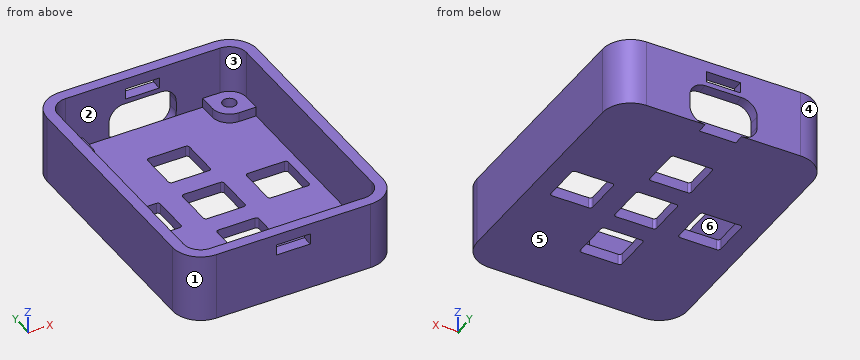
from build123d import *

# Parameters (mm, degrees)
BOX011_W          = 10
BOX011_H          = 3.2
BOX011_DEPTH      = 6.2
FILLET008_R       = 2.29
BOX013_W          = 5
BOX013_H          = 1.6
BOX013_DEPTH      = 1.6
BOX012_W          = 5
BOX012_H          = 1.6
BOX012_DEPTH      = 1.6
BOX009_W          = 6.2
BOX009_H          = 6.2
BOX009_DEPTH      = 2
FILLET004_R       = 0.4
BOX007_W          = 6.2
BOX007_H          = 6.2
BOX007_DEPTH      = 2
FILLET005_R       = 0.4
BOX010_W          = 6.2
BOX010_H          = 6.2
BOX010_DEPTH      = 2
FILLET006_R       = 0.4
BOX006_W          = 6.2
BOX006_H          = 6.2
BOX006_DEPTH      = 2
FILLET007_R       = 0.4
BOX008_W          = 6.2
BOX008_H          = 6.2
BOX008_DEPTH      = 2
FILLET003_R       = 0.4
CYLINDER003_R     = 1
CYLINDER003_DEPTH = 10
CYLINDER002_R     = 1
CYLINDER002_DEPTH = 10
CYLINDER001_R     = 1
CYLINDER001_DEPTH = 10
CYLINDER_R        = 1
CYLINDER_DEPTH    = 10
BOX002_W          = 5.08
BOX002_H          = 5.08
BOX002_DEPTH      = 3
BOX003_W          = 5.08
BOX003_H          = 5.08
BOX003_DEPTH      = 3
BOX004_W          = 5.08
BOX004_H          = 5.08
BOX004_DEPTH      = 3
BOX005_W          = 5.08
BOX005_H          = 5.08
BOX005_DEPTH      = 3
BOX001_W          = 28
BOX001_H          = 38.2
BOX001_DEPTH      = 10
BOX_W             = 31.2
BOX_H             = 41.4
BOX_DEPTH         = 10.1
FILLET_R          = 2.54
FILLET001_R       = 2.54
FILLET002_R       = 4.14


with BuildPart() as led:
    # Box011 → Box011 (new body)
    with BuildSketch(Plane(origin=(9, 38.2, 0), x_dir=(1, 0, 0), z_dir=(0, 0, 1))):
        with Locations((5, 1.6)):
            Rectangle(BOX011_W, BOX011_H)
    extrude(amount=BOX011_DEPTH)

    # Fillet008
    fillet008_edges = [led.edges().sort_by_distance(p)[0] for p in [
        (9, 39.8, 6.2),
        (9, 39.8, 0),
        (19, 39.8, 6.2),
        (19, 39.8, 0),
    ]]
    fillet(fillet008_edges, radius=FILLET008_R)


with BuildPart() as obj1:
    # Box013 → Box013 (new body)
    with BuildSketch(Plane(origin=(11.5, 38.2, 6.9), x_dir=(1, 0, 0), z_dir=(0, 0, 1))):
        with Locations((2.5, 0.8)):
            Rectangle(BOX013_W, BOX013_H)
    extrude(amount=BOX013_DEPTH)


with BuildPart() as nut:
    # Box012 → Box012 (new body)
    with BuildSketch(Plane(origin=(11.5, -1.6, 6.9), x_dir=(1, 0, 0), z_dir=(0, 0, 1))):
        with Locations((2.5, 0.8)):
            Rectangle(BOX012_W, BOX012_H)
    extrude(amount=BOX012_DEPTH)

    # Fusion003: union obj1
    add(obj1.part)


with BuildPart() as fillet004:
    # Box009 → Box009 (new body)
    with BuildSketch(Plane(origin=(1.4, 16.3, 0), x_dir=(1, 0, 0), z_dir=(0, 0, 1))):
        with Locations((3.1, 3.1)):
            Rectangle(BOX009_W, BOX009_H)
    extrude(amount=BOX009_DEPTH)

    # Fillet004
    fillet004_edges = [fillet004.edges().sort_by_distance(p)[0] for p in [
        (1.4, 16.3, 1),
        (1.4, 22.5, 1),
        (7.6, 16.3, 1),
        (7.6, 22.5, 1),
    ]]
    fillet(fillet004_edges, radius=FILLET004_R)


with BuildPart() as fillet005:
    # Box007 → Box007 (new body)
    with BuildSketch(Plane(origin=(10.9, 16.3, 0), x_dir=(1, 0, 0), z_dir=(0, 0, 1))):
        with Locations((3.1, 3.1)):
            Rectangle(BOX007_W, BOX007_H)
    extrude(amount=BOX007_DEPTH)

    # Fillet005
    fillet005_edges = [fillet005.edges().sort_by_distance(p)[0] for p in [
        (10.9, 16.3, 1),
        (10.9, 22.5, 1),
        (17.1, 16.3, 1),
        (17.1, 22.5, 1),
    ]]
    fillet(fillet005_edges, radius=FILLET005_R)


with BuildPart() as fillet006:
    # Box010 → Box010 (new body)
    with BuildSketch(Plane(origin=(20.4, 16.3, 0), x_dir=(1, 0, 0), z_dir=(0, 0, 1))):
        with Locations((3.1, 3.1)):
            Rectangle(BOX010_W, BOX010_H)
    extrude(amount=BOX010_DEPTH)

    # Fillet006
    fillet006_edges = [fillet006.edges().sort_by_distance(p)[0] for p in [
        (20.4, 16.3, 1),
        (20.4, 22.5, 1),
        (26.6, 16.3, 1),
        (26.6, 22.5, 1),
    ]]
    fillet(fillet006_edges, radius=FILLET006_R)


with BuildPart() as fillet007:
    # Box006 → Box006 (new body)
    with BuildSketch(Plane(origin=(10.9, 7.2, 0), x_dir=(1, 0, 0), z_dir=(0, 0, 1))):
        with Locations((3.1, 3.1)):
            Rectangle(BOX006_W, BOX006_H)
    extrude(amount=BOX006_DEPTH)

    # Fillet007
    fillet007_edges = [fillet007.edges().sort_by_distance(p)[0] for p in [
        (10.9, 7.2, 1),
        (10.9, 13.4, 1),
        (17.1, 7.2, 1),
        (17.1, 13.4, 1),
    ]]
    fillet(fillet007_edges, radius=FILLET007_R)


with BuildPart() as buttons:
    # Box008 → Box008 (new body)
    with BuildSketch(Plane(origin=(10.9, 25.5, 0), x_dir=(1, 0, 0), z_dir=(0, 0, 1))):
        with Locations((3.1, 3.1)):
            Rectangle(BOX008_W, BOX008_H)
    extrude(amount=BOX008_DEPTH)

    # Fillet003
    fillet003_edges = [buttons.edges().sort_by_distance(p)[0] for p in [
        (10.9, 25.5, 1),
        (10.9, 31.7, 1),
        (17.1, 25.5, 1),
        (17.1, 31.7, 1),
    ]]
    fillet(fillet003_edges, radius=FILLET003_R)

    # Fusion002: union Fillet004, Fillet005, Fillet006, Fillet007
    add(fillet004.part)
    add(fillet005.part)
    add(fillet006.part)
    add(fillet007.part)


with BuildPart() as zylinder003:
    # Cylinder003 → Cylinder003 (new body)
    with BuildSketch(Plane(origin=(25.46, 35.66, 0.4), x_dir=(1, 0, 0), z_dir=(0, 0, 1))):
        Circle(CYLINDER003_R)
    extrude(amount=CYLINDER003_DEPTH)


with BuildPart() as zylinder002:
    # Cylinder002 → Cylinder002 (new body)
    with BuildSketch(Plane(origin=(2.54, 35.66, 0.4), x_dir=(1, 0, 0), z_dir=(0, 0, 1))):
        Circle(CYLINDER002_R)
    extrude(amount=CYLINDER002_DEPTH)


with BuildPart() as zylinder001:
    # Cylinder001 → Cylinder001 (new body)
    with BuildSketch(Plane(origin=(25.46, 2.54, 0.4), x_dir=(1, 0, 0), z_dir=(0, 0, 1))):
        Circle(CYLINDER001_R)
    extrude(amount=CYLINDER001_DEPTH)


with BuildPart() as fusion001:
    # Cylinder → Cylinder (new body)
    with BuildSketch(Plane(origin=(2.54, 2.54, 0.4), x_dir=(1, 0, 0), z_dir=(0, 0, 1))):
        Circle(CYLINDER_R)
    extrude(amount=CYLINDER_DEPTH)

    # Fusion001: union Zylinder003, Zylinder002, Zylinder001
    add(zylinder003.part)
    add(zylinder002.part)
    add(zylinder001.part)


with BuildPart() as obj2:
    # Box002 → Box002 (new body)
    with BuildSketch(Plane.XY):
        with Locations((2.54, 2.54)):
            Rectangle(BOX002_W, BOX002_H)
    extrude(amount=BOX002_DEPTH)


with BuildPart() as obj3:
    # Box003 → Box003 (new body)
    with BuildSketch(Plane(origin=(22.92, 0, 0), x_dir=(1, 0, 0), z_dir=(0, 0, 1))):
        with Locations((2.54, 2.54)):
            Rectangle(BOX003_W, BOX003_H)
    extrude(amount=BOX003_DEPTH)


with BuildPart() as obj4:
    # Box004 → Box004 (new body)
    with BuildSketch(Plane(origin=(0, 33.12, 0), x_dir=(1, 0, 0), z_dir=(0, 0, 1))):
        with Locations((2.54, 2.54)):
            Rectangle(BOX004_W, BOX004_H)
    extrude(amount=BOX004_DEPTH)


with BuildPart() as obj5:
    # Box005 → Box005 (new body)
    with BuildSketch(Plane(origin=(22.92, 33.12, 0), x_dir=(1, 0, 0), z_dir=(0, 0, 1))):
        with Locations((2.54, 2.54)):
            Rectangle(BOX005_W, BOX005_H)
    extrude(amount=BOX005_DEPTH)


with BuildPart() as obj6:
    # Box001 → Box001 (new body)
    with BuildSketch(Plane.XY.offset(1.6)):
        with Locations((14, 19.1)):
            Rectangle(BOX001_W, BOX001_H)
    extrude(amount=BOX001_DEPTH)


with BuildPart() as cut005:
    # Box → Box (new body)
    with BuildSketch(Plane(origin=(-1.6, -1.6, 0), x_dir=(1, 0, 0), z_dir=(0, 0, 1))):
        with Locations((15.6, 20.7)):
            Rectangle(BOX_W, BOX_H)
    extrude(amount=BOX_DEPTH)

    # Cut: cut obj6
    add(obj6.part, mode=Mode.SUBTRACT)

    # Fusion: union obj2, obj3, obj4, obj5
    add(obj2.part)
    add(obj3.part)
    add(obj4.part)
    add(obj5.part)

    # Fillet
    fillet_edges = [cut005.edges().sort_by_distance(p)[0] for p in [
        (22.92, 33.12, 2.3),
        (22.92, 5.08, 2.3),
        (5.08, 33.12, 2.3),
        (5.08, 5.08, 2.3),
    ]]
    fillet(fillet_edges, radius=FILLET_R)

    # Fillet001
    fillet001_edges = [cut005.edges().sort_by_distance(p)[0] for p in [
        (28, 38.2, 6.55),
        (0, 38.2, 6.55),
        (28, 0, 6.55),
        (0, 0, 6.55),
    ]]
    fillet(fillet001_edges, radius=FILLET001_R)

    # Fillet002
    fillet002_edges = [cut005.edges().sort_by_distance(p)[0] for p in [
        (-1.6, -1.6, 5.05),
        (-1.6, 39.8, 5.05),
        (29.6, 39.8, 5.05),
        (29.6, -1.6, 5.05),
    ]]
    fillet(fillet002_edges, radius=FILLET002_R)

    # Cut001: cut Fusion001
    add(fusion001.part, mode=Mode.SUBTRACT)

    # Cut003: cut Buttons
    add(buttons.part, mode=Mode.SUBTRACT)

    # Cut004: cut Nut
    add(nut.part, mode=Mode.SUBTRACT)

    # Cut005: cut LED
    add(led.part, mode=Mode.SUBTRACT)


solid = cut005.part
The model under review builds one solid part; all positions refer to its coordinate system, in mm. Face numbers are marked on the shaded views. A direction names the side the tool comes from. Coordinates: 2 decimals unless noted, no trailing zeros. Write each loop counter-clockwise with the first axis right and the second up, starting at its lowest first coordinate (ties: lowest second). Pieces come first, ordered by that corner, then holes. Notation, with made-up numbers: (-14.5, 53) - (0.5, 53) arc R8 ccw to (0.5, 60) - close; hole circle Ø9 at (58.25, 53). An arc over 180 degrees is marked (long way). Answer as a JSON object with one key per item and string values. Group by question number.
1. Add section A-A (x = 12.5). Give the number of separate pieces and of enclosed holes in the cut face, plus the area to 3 significant figures.
2. Add section B-B (y = 10.5). Give the boundary of the cut face in (x, z).
3. Add section C-C (x = 21.5). Give the boundary of the cut face in (y, z), plus the area to 3 significant figures.
4. To check wall thickness, follow probe 1 along Y at (x, z) = (25.46, 1.1); probe 2 along Y at (x, z) = (25.46, 1.9); probe 3 along X at (y, z) = (34.5, 5). State the ranges of each line that lie inside material, in increasing order.
5. Mouldability with a two-part tool opening along X and no side actions: class the marked faces 3, 4, 5 and 6 as pulls with the +X half, pulls with the -X half, needs draft (parallel to the pull), parting line crosses it, or undercut.
6. Machinability: for the marked faces 1 and 2, which of the approach directions +Z, -Z, +X, -X, +Y, -Y give a long, thin tool a straight path to every point of the face, cutting with its end or side? Answer none if there is none.
7. Add section D-D (z = 8). Give the boundary of the cut face in (x, y), plus the area to 3 significant figures.
8. Clearance check with flat-ended pins moving along their axes: pin 1 Ø1.6 at (x, y) = (2.5, 36) entering from +Z; pin 2 Ø6 at (x, y) = (11.5, 23.5) entering from +Z; pin 3 Ø0.7 at (y, z) = (37.5, 2) entering from +X; pin 4 Ø1.5 at (x, y) = (24, 20.5) entering from +Z. State where each tip first meets the part, or that it passes through.
Findings:
{
 "1": {"separate pieces": "7", "enclosed holes": "0", "area": "48.6 mm²"},
 "2": {"outline": "(-1.6, 0) - (10.9, 0) - (10.9, 1.6) - (0, 1.6) - (0, 10.1) - (-1.6, 10.1) - close; (17.1, 0) - (29.6, 0) - (29.6, 10.1) - (28, 10.1) - (28, 1.6) - (17.1, 1.6) - close"},
 "3": {"outline": "(-1.6, 0) - (16.3, 0) - (16.3, 1.6) - (0, 1.6) - (0, 10.1) - (-1.6, 10.1) - close; (22.5, 0) - (39.8, 0) - (39.8, 10.1) - (38.2, 10.1) - (38.2, 1.6) - (22.5, 1.6) - close", "area": "83.5 mm²"},
 "4": {"probe 1": "-1.6 to 1.54, 3.54 to 16.3, 22.5 to 34.66, 36.66 to 39.8", "probe 2": "-1.6 to 1.54, 3.54 to 5.08, 33.12 to 34.66, 36.66 to 39.8", "probe 3": "-1.6 to 0, 28 to 29.6"},
 "5": {"face 3": "undercut", "face 4": "pulls with the -X half", "face 5": "needs draft", "face 6": "undercut"},
 "6": {"face 1": "+Z, -Z, -X, -Y", "face 2": "+Z"},
 "7": {"outline": "(-1.6, 2.54) arc R4.14 ccw to (2.54, -1.6) - (11.5, -1.6) - (11.5, 0) - (2.54, 0) arc R2.54 cw to (0, 2.54) - (0, 35.66) arc R2.54 cw to (2.54, 38.2) - (11.5, 38.2) - (11.5, 39.8) - (2.54, 39.8) arc R4.14 ccw to (-1.6, 35.66) - close; (16.5, -1.6) - (25.46, -1.6) arc R4.14 ccw to (29.6, 2.54) - (29.6, 35.66) arc R4.14 ccw to (25.46, 39.8) - (16.5, 39.8) - (16.5, 38.2) - (25.46, 38.2) arc R2.54 cw to (28, 35.66) - (28, 2.54) arc R2.54 cw to (25.46, 0) - (16.5, 0) - close", "area": "197 mm²"},
 "8": {"pin 1": "z = 3", "pin 2": "z = 1.6", "pin 3": "x = 29.32", "pin 4": "through"}
}
